For this review, take the finished solid that the model builds, in its own axes (mm). Coordinates: 2 decimals unless noted, no trailing zeros. Loops run counter-clockwise (first coordinate to the right, second up) from the corner with the lowest first, then second, coordinate; pieces in that order, holes last. Notation, with made-up numbers: M -31.5,-29 L -1.5,-29 A31 ccw -1.5,-1 Z; hole C -3.5,53.25 d6. An arc over 180 degrees is marked long. Answer as a JSON object with one key per item and string values. Group by question number.
Item 1: Add section B-B (z = -42.5). State the section outline as (x, y) points.
Item 2: Add section C-C (x = -1.8). State the section outline as (y, z) points, then the cut area to 3 significant figures.
Item 3: Wall thickness on L1, parallel to Y at x = -0.9, z = -240.5; L2, parallel to Z at x = 1.1, y = 15.5; L3, parallel to Z at x = 0.15, y = 13: over which ranges is each line inside the solid? List them lowest first. Write a range as from..to.
Item 4: Add section A-A (y = 0). State the section outline as (x, z) points, then the cut area to 3 significant figures.
Item 5: Insertion check: pin 1 (1.5 mm diameter, centred on x = 0, y = 18, fed in from -Z); pin 2 (3 mm diameter, centred on x = 0.5, y = 16, fed in from +Z); pin 3 (3 mm diameter, centred on x = -0.5, z = 180.5, fed in from +Y). Each pin has a flat end and moves straight along its axis. Give the tip position at first contact, or say it passes through.
from build123d import *

# Parameters (mm, degrees)
RESSALTO_EXTRUS_O1_DEPTH = 3
BOSS_EXTRUDE1_DEPTH      = 3
CUT_EXTRUDE1_DEPTH       = 291.521948294
FILLET1_R                = 5
FILLET2_R                = 3.5


with BuildPart() as part:
    # Esboço1 → Ressalto-extrusão1 (new, symmetric)
    with BuildSketch(Plane(origin=(0, 0, 0), x_dir=(0, 0, -1), z_dir=(1, 0, 0))):
        with BuildLine():
            Line((-281.89, 7.7), (281.89, 7.7))
            ThreePointArc((281.89, 7.7), (289.59, 0), (281.89, -7.7))
            Line((281.89, -7.7), (-281.89, -7.7))
            ThreePointArc((-281.89, -7.7), (-289.59, 0), (-281.89, 7.7))
        make_face()
        with BuildLine():
            Line((-281.89, 6.2), (281.89, 6.2))
            ThreePointArc((281.89, 6.2), (288.09, 0), (281.89, -6.2))
            Line((281.89, -6.2), (-281.89, -6.2))
            ThreePointArc((-281.89, -6.2), (-288.09, 0), (-281.89, 6.2))
        make_face(mode=Mode.SUBTRACT)
    extrude(amount=RESSALTO_EXTRUS_O1_DEPTH, both=True)

    # Sketch1 → Boss-Extrude1 (add, symmetric)
    with BuildSketch(Plane(origin=(0, 0, 0), x_dir=(0, 0, -1), z_dir=(1, 0, 0))):
        Polygon((26.184631905, 14.464067762), (26.184631905, 11.464067762), (31.684631905, 6.2), (33.854011297, 6.2), (27.684631905, 12.104732939), (27.684631905, 14.464067762), (27.684631905, 22.464067762), (26.184631905, 22.464067762), align=None)
        Polygon((-24.815368095, 11.464067762), (-24.815368095, 14.464067762), (-24.815368095, 22.464067762), (-26.315368095, 22.464067762), (-26.315368095, 14.464067762), (-26.315368095, 12.104732939), (-32.484747486, 6.2), (-30.315368095, 6.2), align=None)
    extrude(amount=BOSS_EXTRUDE1_DEPTH, both=True)

    # Sketch2 → Cut-Extrude1 (cut, through all)
    with BuildSketch(Plane(origin=(3, 0, 0), x_dir=(0, 0, -1), z_dir=(1, 0, 0))):
        Polygon((-30.315368095, 6.2), (-28.748139029, 7.7), (30.117402839, 7.7), (31.684631905, 6.2), align=None)
    extrude(amount=-CUT_EXTRUDE1_DEPTH, mode=Mode.SUBTRACT)

    # Fillet1
    fillet1_edges = [part.edges().sort_by_distance(p)[0] for p in [
        (0, 11.464067762, -26.184631905),
        (0, 6.2, -31.684631905),
        (0, 6.2, 30.315368095),
        (0, 11.464067762, 24.815368095),
    ]]
    fillet(fillet1_edges, radius=FILLET1_R)

    # Fillet2
    fillet2_edges = [part.edges().sort_by_distance(p)[0] for p in [
        (0, 12.104732939, 26.315368095),
        (0, 7.7, 30.917518421),
        (0, 7.7, -32.286782231),
        (0, 12.104732939, -27.684631905),
    ]]
    fillet(fillet2_edges, radius=FILLET2_R)


solid = part.part
From the geometry:
{
 "1": {"outline": "M -3,-7.7 L 3,-7.7 L 3,-6.2 L -3,-6.2 Z; M -3,6.2 L 3,6.2 L 3,7.7 L -3,7.7 Z"},
 "2": {"outline": "M -7.7,-281.89 A7.7 ccw 7.7,-281.89 L 7.7,-33.69 A3.5 cw 8.67,-31.27 L 11.07,-28.76 A3.5 cw 13.6,-27.68 L 22.46,-27.68 L 22.46,-26.18 L 13.6,-26.18 A5 ccw 9.99,-27.73 L 7.59,-30.23 A5 ccw 6.2,-33.69 L 6.2,-281.89 A6.2 cw -6.2,-281.89 L -6.2,281.89 A6.2 cw 6.2,281.89 L 6.2,32.32 A5 ccw 7.59,28.87 L 9.99,26.36 A5 ccw 13.6,24.82 L 22.46,24.82 L 22.46,26.32 L 13.6,26.32 A3.5 cw 11.07,27.4 L 8.67,29.9 A3.5 cw 7.7,32.32 L 7.7,281.89 A7.7 ccw -7.7,281.89 Z", "area": "1,710 mm²"},
 "3": {"L1": "y = -7.7..-6.2, 6.2..7.7", "L2": "z = -27.68..-26.18, 24.82..26.32", "L3": "z = -27.74..-26.22, 24.85..26.37"},
 "4": {"outline": "M -3,-289.59 L 3,-289.59 L 3,-288.09 L -3,-288.09 Z; M -3,288.09 L 3,288.09 L 3,289.59 L -3,289.59 Z", "area": "18.0 mm²"},
 "5": {"pin 1": "stops at z = -27.68", "pin 2": "stops at z = 26.32", "pin 3": "stops at y = 7.7"}
}
